from build123d import *

# Parameters (mm, degrees)
F0_W     = 5.2
F0_H     = 5.2
F0_W_2   = 5.1
F0_H_2   = 5.1
F0_R     = 3.1
F0_R_2   = 3.05
F1_DEPTH = 2


with BuildPart() as f1:
    # F0 (on Top) → F1 (new body)
    with BuildSketch(Plane.XY):
        with BuildLine():
            Line((-17.674136, 4.078372), (-44.748526, 4.078372))
            Line((-44.748526, 4.078372), (-44.748526, -4.046109))
            Line((-44.748526, -4.046109), (-17.674136, -4.046109))
            ThreePointArc((-17.674136, -4.046109), (-15.694237, -3.226008), (-14.874136, -1.246109))
            Line((-14.874136, -1.246109), (-14.874136, 1.278372))
            ThreePointArc((-14.874136, 1.278372), (-15.694237, 3.258271), (-17.674136, 4.078372))
        make_face()
        with Locations((-40.60166, 0)):
            Rectangle(F0_W, F0_H, mode=Mode.SUBTRACT)
        with Locations((-33.513274, 0)):
            Rectangle(F0_W_2, F0_H_2, mode=Mode.SUBTRACT)
        with Locations((-26.299188, 0)):
            Circle(F0_R, mode=Mode.SUBTRACT)
        with Locations((-18.936377, 0)):
            Circle(F0_R_2, mode=Mode.SUBTRACT)
    extrude(amount=F1_DEPTH)


solid = f1.part
The model under review builds one solid part; all positions refer to its coordinate system, in mm. A direction names the side the tool comes from. Coordinates: 2 decimals unless noted, no trailing zeros. Write each loop counter-clockwise with the first axis right and the second up, starting at its lowest first coordinate (ties: lowest second). Pieces come first, ordered by that corner, then holes. Notation, with made-up numbers: (27, -0.5) - (69, -0.5) arc R20 cw to (69, 8.5) - close; hole circle Ø1 at (-29.5, 86). An arc over 180 degrees is marked (long way). Answer as a JSON object with one key per item and string values. Group by question number.
1. Machinability: for faces 4 (the face through (-30.963, 0, 1)), 5 (the face through (-44.749, 0, 1)), which of the approach directions +Z, -Z, +X, -X, +Y, -Y give a long, thin tool a straight path to every point of the face, cutting with its end or side? Answer none if there is none.
2. Add section B-B (y = 0). Give the boundary of the cut face in (x, z), plus the area to 3 significant figures.
3. Add section D-D (x = -18.5). Give the boundary of the cut face in (y, z).
4. Add section C-C (z = 1.45). Give the boundary of the cut face in (x, y), plus the area to 3 significant figures.
5. Add section A-A (x = -42). Give the boundary of the cut face in (y, z), plus the area to 3 significant figures.
6. To check wall thickness, follow probe 1 along Y at (x, z) = (-42.75, 0.9); probe 2 along X at (y, z) = (2, 0.75); probe 3 along X at (y, z) = (1, 1.75). State the ranges of each line that lie inside material, in increasing order.
7. Mouldability with a two-part tool opening along X and no side actions: class faces 1 (the face through (-15.72, -3.25, 0.99)), 2 (the face through (-43.202, 0, 1)), 3 (the face through (-30, 0, 0)) as pulls with the +X half, pulls with the -X half, needs draft (parallel to the pull), parting line crosses it, or undercut.
Findings:
{
 "1": {"face 4": "+Z, -Z", "face 5": "+Z, -Z, -X, +Y, -Y"},
 "2": {"outline": "(-44.75, 0) - (-43.2, 0) - (-43.2, 2) - (-44.75, 2) - close; (-38, 0) - (-36.06, 0) - (-36.06, 2) - (-38, 2) - close; (-30.96, 0) - (-29.4, 0) - (-29.4, 2) - (-30.96, 2) - close; (-23.2, 0) - (-21.99, 0) - (-21.99, 2) - (-23.2, 2) - close; (-15.89, 0) - (-14.87, 0) - (-14.87, 2) - (-15.89, 2) - close", "area": "14.5 mm²"},
 "3": {"outline": "(-4.05, 0) - (-3.02, 0) - (-3.02, 2) - (-4.05, 2) - close; (3.02, 0) - (4.08, 0) - (4.08, 2) - (3.02, 2) - close"},
 "4": {"outline": "(-44.75, -4.05) - (-17.67, -4.05) arc R2.8 ccw to (-14.87, -1.25) - (-14.87, 1.28) arc R2.8 ccw to (-17.67, 4.08) - (-44.75, 4.08) - close; hole (-43.2, -2.6) - (-38, -2.6) - (-38, 2.6) - (-43.2, 2.6) - close; hole (-36.06, -2.55) - (-30.96, -2.55) - (-30.96, 2.55) - (-36.06, 2.55) - close; hole circle Ø6.2 at (-26.3, 0); hole circle Ø6.1 at (-18.94, 0)", "area": "127 mm²"},
 "5": {"outline": "(-4.05, 0) - (-2.6, 0) - (-2.6, 2) - (-4.05, 2) - close; (2.6, 0) - (4.08, 0) - (4.08, 2) - (2.6, 2) - close", "area": "5.85 mm²"},
 "6": {"probe 1": "-4.05 to -2.6, 2.6 to 4.08", "probe 2": "-44.75 to -43.2, -38 to -36.06, -30.96 to -28.67, -23.93 to -21.24, -16.63 to -14.97", "probe 3": "-44.75 to -43.2, -38 to -36.06, -30.96 to -29.23, -23.36 to -21.82, -16.05 to -14.87"},
 "7": {"face 1": "pulls with the +X half", "face 2": "undercut", "face 3": "needs draft"}
}
